```python
from build123d import *

# Parameters (mm, degrees)
F0_W     = 50
F0_H     = 50
F0_R     = 12.5
F1_DEPTH = 25
F3_DEPTH = 25
F5_DEPTH = 50
F7_DEPTH = 25


with BuildPart() as f1:
    # F0 (on Front) → F1 (new body)
    with BuildSketch(Plane.XZ):
        Rectangle(F0_W, F0_H)
        Circle(F0_R, mode=Mode.SUBTRACT)
    extrude(amount=F1_DEPTH)

    # F2 (on face) → F3 (join)
    with BuildSketch(Plane.XZ.offset(25)):
        with BuildLine():
            Line((-8.8388347648, -8.8388347648), (-25, -25))
            Line((-25, -25), (25, -25))
            Line((25, -25), (25, 25))
            Line((25, 25), (8.8388347648, 8.8388347648))
            ThreePointArc((8.8388347648, 8.8388347648), (11.5484941564, 4.7835429046), (12.5, 0))
            ThreePointArc((12.5, 0), (4.7835429046, -11.5484941564), (-8.8388347648, -8.8388347648))
        make_face()
    extrude(amount=F3_DEPTH)

    # F4 (on face) → F5 (cut)
    with BuildSketch(Plane(origin=(0, 0, 0), x_dir=(0, -1, 0), z_dir=(-0.7071067812, 0, 0.7071067812))):
        Polygon((40.7957995796, -31.3931250338), (40.7957995796, -19.3931250338), (30.4034947342, -25.3931250338), align=None)
        Polygon((42.8262037943, 21.4346205463), (42.8262037943, 27.7791293861), (37.3316979645, 30.951383806), (31.8371921347, 27.7791293861), (31.8371921347, 21.4346205463), (37.3316979645, 18.2623661264), align=None)
    extrude(amount=-F5_DEPTH, mode=Mode.SUBTRACT)

    # F6 (on face) → F7 (join)
    with BuildSketch(Plane.XZ.offset(25)):
        Polygon((-11.8569600062, 19.0248098224), (-18.7698883339, 19.0248098224), (-22.2263524977, 13.0380382761), (-18.7698883339, 7.0512667298), (-11.8569600062, 7.0512667298), (-8.4004958423, 13.0380382761), align=None)
    extrude(amount=F7_DEPTH)


solid = f1.part
```
Work out the finished part from the listing and answer in its coordinate system (mm). A direction names the side the tool comes from. Round coordinates to 2 decimals unless told otherwise and drop trailing zeros. Loops run counter-clockwise (first coordinate to the right, second up) from the corner with the lowest first, then second, coordinate; pieces in that order, holes last.
(1) The part is cut by section A-A, the plane x = 0. Give the vertices of the cut face in (y, z).
Computed values:
outline: (-50, -25) - (0, -25) - (0, -12.5) - (-50, -12.5) - close; (-25, 12.5) - (0, 12.5) - (0, 25) - (-25, 25) - close
(2) Each of these flat-tipped pins is pushed along its axis until it touches: P1, Ø15, axis at x = 0, z = 0, coming from the -Y side; P2, Ø10, axis at x = -13.5, z = -5, coming from the -Y side; P3, Ø3.5, axis at x = -15.5, y = -36, coming from the +Z side. Where does it stop, or does it pass through?
Computed values:
P1: passes through
P2: stops at y = -25
P3: stops at z = 19.02
(3) For faces 5 (the flat face through (17, -43, 17)), 6 (the flat face through (-20.522, -37.325, 10.087)), 7 (the flat face through (-5.9, -25, 11.5)), 8 (the flat face through (-20.474, -37.325, 16.073)), 9 (the flat face through (21, -42.826, 14)), determine the directions among +Z, -Z, +X, -X, +Y, -Y from which every point of the face is accessible in a straight line to the end or side of a thin tool.
Computed values:
face 5: +Z, -Y
face 6: -X, -Y
face 7: -Y
face 8: +Z, -X, -Y
face 9: none
(4) The part is cut by section B-B, the plane y = -21. Give the vertices of the cut face in (x, z), and give its area (3 significant figures).
Computed values:
outline: (-25, -25) - (25, -25) - (25, 25) - (-25, 25) - close; hole circle Ø25 at (0, 0)
area: 2,010 mm2
(5) The mould has two halves that part along X. Classify faces 1 (the flat face through (11, -50, -11)), 2 (the flat face through (-16.886, -34.372, -22.266)), 3 (the flat face through (-15, -37, -15)), 4 (the flat face through (25, -25, 0)): pulls with the +X half, pulls with the -X half, needs draft (parallel to the pull), parting line crosses it, or undercut.
Computed values:
face 1: needs draft
face 2: undercut
face 3: pulls with the -X half
face 4: pulls with the +X half
(6) Find the intervals of material crossed by L1, parallel to X at y = -11.25, z = 0; L2, parallel to Y at x = -18.5, z = 6.5, in increasing order.
Computed values:
L1: x = -25 to -12.5, 12.5 to 25
L2: y = -25 to 0
(7) The part is cut by section C-C, the plane z = 3. Give the vertices of the cut face in (x, y).
Computed values:
outline: (-25, -25) - (-12.13, -25) - (-12.13, 0) - (-25, 0) - close; (12.13, -50) - (25, -50) - (25, -39.99) - (22.83, -37.33) - (25, -34.67) - (25, 0) - (12.13, 0) - close
(8) The part is cut by section D-D, the plane y = -45.5. Give the vertices of the cut face in (x, z), and give its area (3 significant figures).
Computed values:
outline: (-25, -25) - (25, -25) - (25, 25) - (8.84, 8.84) arc R12.5 cw to (-8.84, -8.84) - close; (-22.23, 13.04) - (-18.77, 7.05) - (-11.86, 7.05) - (-8.4, 13.04) - (-11.86, 19.02) - (-18.77, 19.02) - close
area: 1,130 mm2
